Can you work these out from the drawing? Everything is in mm from the part's minimum corner. A direction names the side the tool comes from. Round coordinates to 2 decimals unless told otherwise and drop trailing zeros. Order: outer loops, then holes, each group sorted by start corner. A loop starts at its lowest first (then second) coordinate and runs counter-clockwise, first axis right, second up. Notation, with made-up numbers: M 71,-13 L 109,-13 A30 cw 109,24 Z; hole C 63.25,-12.75 d1. An arc over 180 degrees is marked long. Write item = value, one per line. Start each with the question number.
Item 1: I'm going to push a flat-ended pin straight in: P1, Ø10, axis at x = 55, z = 42.5, coming from the -Y side. Where does the tip first touch, or does it pass through?
Item 2: I want a section at D-D, the plane z = 36. List the corners of the cut face in (x, y) for me (1 decimal).
Item 3: Please list where these lines run through material, in increasing order: L1, parallel to Z at x = 15.5, y = 63; L2, parallel to Z at x = 58, y = 36; L3, parallel to X at y = 36, z = 31 (1 decimal).
Item 4: I want a section at C-C, the plane x = 87. List the corners of the cut face in (y, z) for me, plus the area to 3 significant figures.
Item 5: I want a section at A-A, the plane y = 32. List the corners of the cut face in (x, z) for me.
Item 6: For the marked faces 1 and 2, which set-ups out of +Z, -Z, +X, -X, +Y, -Y let a thin tool reach every point of the face, with its end or its side?
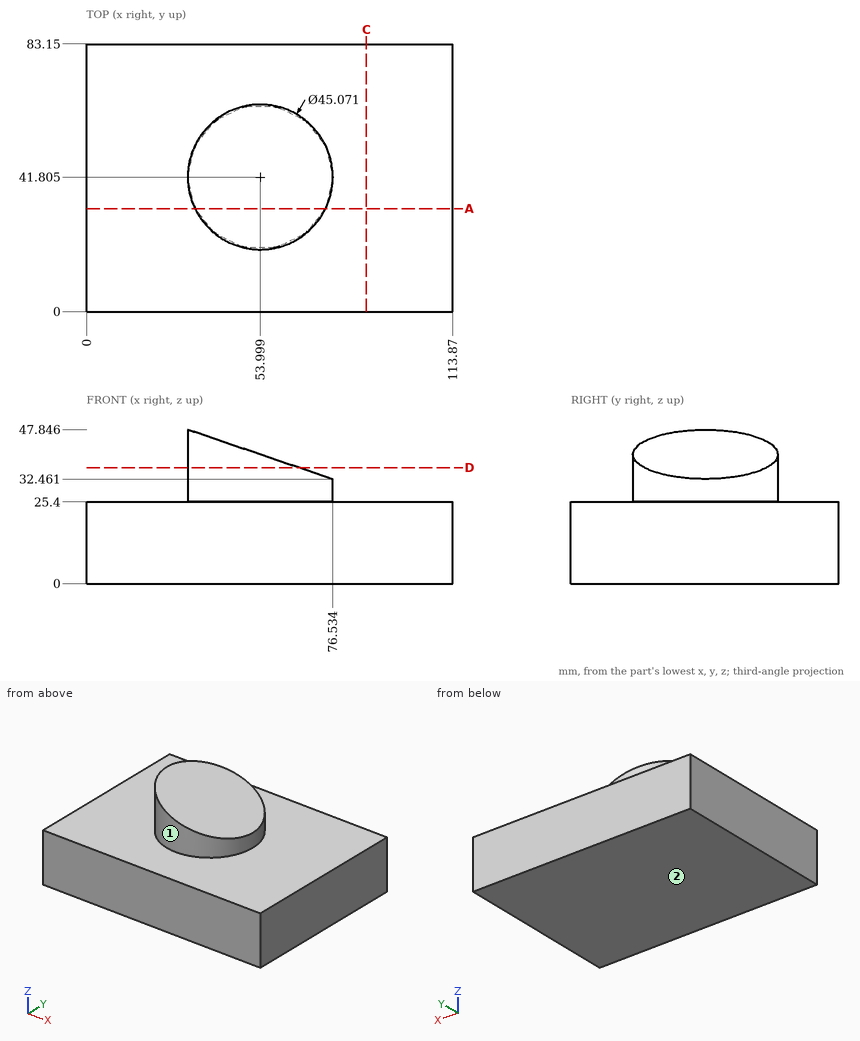
Filled in:
q1.P1 = 19.27
q2.outline = M 66.2,22.8 L 66.2,60.8 A22.5 ccw long Z
q3.L1 = 0 to 25.4
q3.L2 = 0 to 38.79
q3.L3 = 32.2 to 75.8
q4.outline = M 0,0 L 83.15,0 L 83.15,25.4 L 0,25.4 Z
q4.area = 2,110 mm^2
q5.outline = M 0,0 L 113.87,0 L 113.87,25.4 L 74.29,25.4 L 74.29,33.23 L 33.71,47.08 L 33.71,25.4 L 0,25.4 Z
q6.face_1 = +Z
q6.face_2 = -Z, +X, -X, +Y, -Y
